Can you work these out from the drawing? Everything is in mm from the part's minimum corner. A direction names the side the tool comes from. Coordinates: 2 decimals unless noted, no trailing zeros. Order: outer loops, then holes, each group sorted by start corner. A loop starts at its lowest first (then second) coordinate and runs counter-clockwise, first axis right, second up. Notation, with made-up numbers: (30.25, 46.5) - (81.25, 46.5) arc R19 ccw to (81.25, 74.5) - close; hole circle Ø11 at (58, 80.25). An arc over 180 degrees is marked (long way). Answer as CSV lines item,"result". Start each with the question number.
Q1. Suppose I cut it at A-A (z = 23). Please give me the cut outline in (x, y).
Q2. For pin 1 Ø1.5 at (x, z) = (48.5, 130) entering from -Y; pin 2 Ø10 at (x, z) = (66.5, 116) entering from +Y; pin 3 Ø1 at (x, y) = (47.5, 39) entering from +Z, each with a flat end and sliding along its axis, tell me the tip position at first contact or that it passes through.
Q3. Suppose I cut it at B-B (y = 30). Please give me the cut outline in (x, z).
Q4. Suppose I cut it at C-C (x = 77). Please give me the cut outline in (y, z), then the cut area to 3 significant figures.
Q5. Suppose I cut it at D-D (y = 14.5). Please give me the cut outline in (x, z).
Q6. For the marked faces 4 and 5, which set-ups out of +Z, -Z, +X, -X, +Y, -Y let a thin tool reach every point of the face, with its end or its side?
Q7. Thinking about a two-plate mould opening in X: for the marked faces 1, 2 and 3, which applies, released by +X, released by -X, zero draft, split by the parting line, or undercut?
Q8. I need wall thicknesses on line 1 (X direction, y = 11, z = 146.5); line 2 (Y direction, x = 156, z = 23); line 3 (Z direction, x = 135, y = 33) (1 decimal). Which ranges of each line are inside material? Lowest first, please.
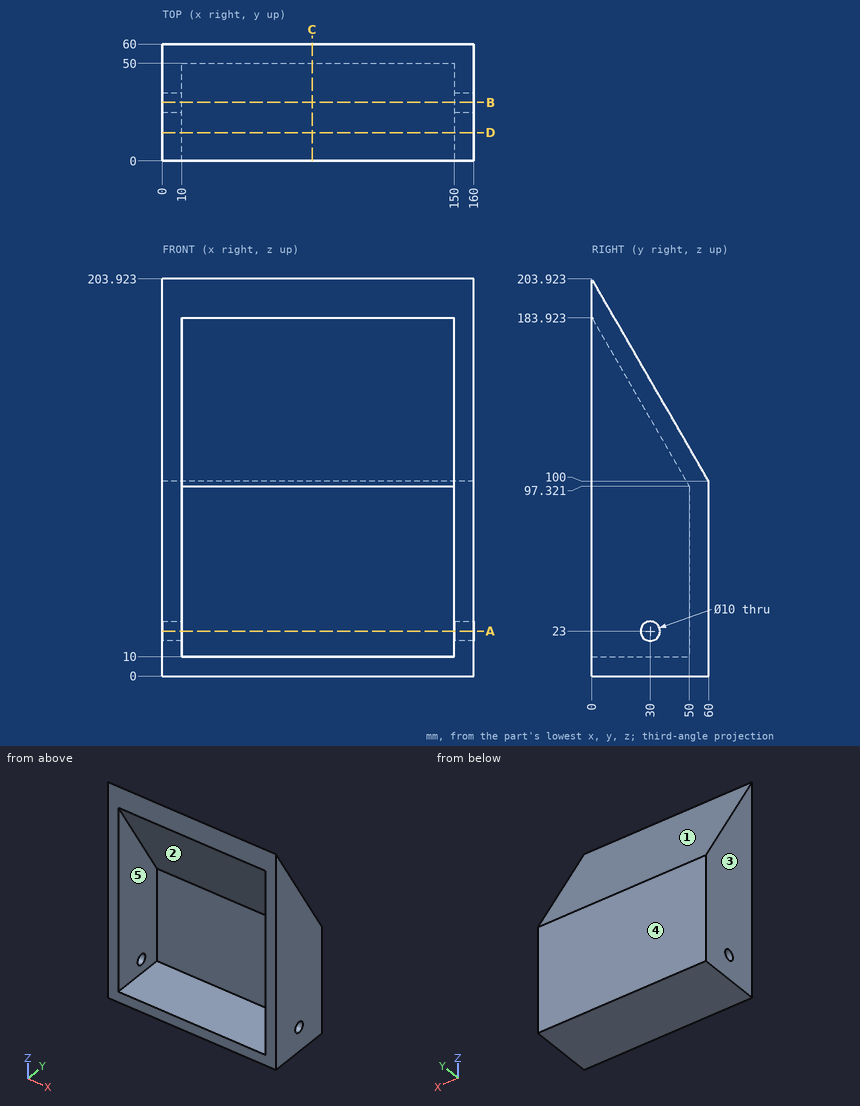
Here are the results:
1,outline,"(0, 0) - (10, 0) - (10, 25) - (0, 25) - close; (0, 35) - (10, 35) - (10, 50) - (150, 50) - (150, 35) - (160, 35) - (160, 60) - (0, 60) - close; (150, 0) - (160, 0) - (160, 25) - (150, 25) - close"
2,pin 1,"stops at y = 30.7"
2,pin 2,"stops at y = 53.65"
2,pin 3,"stops at z = 137.24"
3,outline,"(0, 0) - (160, 0) - (160, 18) - (150, 18) - (150, 10) - (10, 10) - (10, 18) - (0, 18) - close; (0, 28) - (10, 28) - (10, 131.96) - (150, 131.96) - (150, 28) - (160, 28) - (160, 151.96) - (0, 151.96) - close"
4,outline,"(0, 0) - (60, 0) - (60, 100) - (0, 203.92) - (0, 183.92) - (50, 97.32) - (50, 10) - (0, 10) - close"
4,area,"2,590 mm²"
5,outline,"(0, 0) - (160, 0) - (160, 178.81) - (0, 178.81) - close; hole (10, 10) - (150, 10) - (150, 158.81) - (10, 158.81) - close"
6,face 4,"+Z, -Z, +X, -X, +Y"
6,face 5,"-Y"
7,face 1,"zero draft"
7,face 2,"undercut"
7,face 3,"released by -X"
8,line 1,"x = 0 to 10, 150 to 160"
8,line 2,"y = 0 to 25, 35 to 60"
8,line 3,"z = 0 to 10, 126.8 to 146.8"
